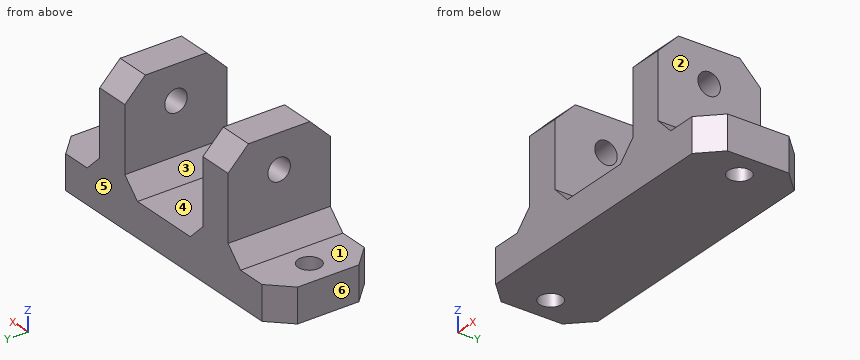
```python
from build123d import *

# Parameters (mm, degrees)
SKETCH_W        = 90
SKETCH_H        = 30
PAD_DEPTH       = 10
SKETCH001_W     = 10
SKETCH001_H     = 30
PAD001_DEPTH    = 30
CHAMFER_SIZE    = 6
SKETCH002_R     = 3.3
HOLE_DEPTH      = 58.01716
HOLE_TIPS_R     = 3.3
CHAMFER001_SIZE = 5
SKETCH003_R     = 3.3
HOLE001_DEPTH   = 25


with BuildPart() as part:
    # Sketch → Pad (new body)
    with BuildSketch(Plane.XY):
        Rectangle(SKETCH_W, SKETCH_H)
    extrude(amount=PAD_DEPTH)

    # Sketch001 → Pad001 (join)
    with BuildSketch(Plane.XY.offset(10)):
        with Locations((20.5, 0)):
            Rectangle(SKETCH001_W, SKETCH001_H)
        with Locations((-20.5, 0)):
            Rectangle(SKETCH001_W, SKETCH001_H)
    extrude(amount=PAD001_DEPTH)

    # Chamfer
    chamfer_edges = [part.edges().sort_by_distance(p)[0] for p in [
        (-45, 15, 5),
        (-45, -15, 5),
        (-20.5, 15, 40),
        (-20.5, -15, 40),
        (20.5, 15, 40),
        (45, 15, 5),
        (20.5, -15, 40),
        (45, -15, 5),
    ]]
    chamfer(chamfer_edges, length=CHAMFER_SIZE)

    # Sketch002 (on Face15 of Chamfer) → Hole (cut)
    with BuildSketch(Plane(origin=(-25.5, 0, 0), x_dir=(0, -1, 0), z_dir=(-1, 0, 0))):
        with Locations((0, 30)):
            Circle(SKETCH002_R)
    extrude(amount=-HOLE_DEPTH, mode=Mode.SUBTRACT)

    # Hole tips → Hole tip 1 section 0
    with BuildSketch(Plane(origin=(32.51716, 0, 0), x_dir=(0, -1, 0), z_dir=(-1, 0, 0)), mode=Mode.PRIVATE) as hole_tip_1_s0:
        with Locations((0, 30)):
            Circle(HOLE_TIPS_R)
    loft([hole_tip_1_s0.sketch, Vertex(34.5, 0, 30)], mode=Mode.SUBTRACT)

    # Chamfer001
    chamfer001_edges = [part.edges().sort_by_distance(p)[0] for p in [
        (25.5, 0, 10),
        (-15.5, 0, 10),
        (-25.5, 0, 10),
        (15.5, 0, 10),
    ]]
    chamfer(chamfer001_edges, length=CHAMFER001_SIZE)

    # Sketch003 (on Face2 of Chamfer001) → Hole001 (cut)
    with BuildSketch(Plane.XY.offset(10)):
        with Locations((-37.5, 0)):
            Circle(SKETCH003_R)
        with Locations((37.5, 0)):
            Circle(SKETCH003_R)
    extrude(amount=-HOLE001_DEPTH, mode=Mode.SUBTRACT)


solid = part.part
```
The model under review builds one solid part; all positions refer to its coordinate system, in mm. Face numbers are marked on the shaded views. A direction names the side the tool comes from. Round coordinates to 2 decimals unless told otherwise and drop trailing zeros. Loops run counter-clockwise (first coordinate to the right, second up) from the corner with the lowest first, then second, coordinate; pieces in that order, holes last. Notation, with made-up numbers: (43.25, -32) -> (70.25, -32) arc R21 cw to (70.25, -15) -> close; hole circle Ø9 at (83, -25.5). An arc over 180 degrees is marked (long way). Answer in a Markdown table with one row per item.
1) Consider section A-A, the plane x = 37.5. Write out the cut boundary in (y, z).
Taken from the geometry:
| item | result |
|---|---|
| outline | (-15, 0) -> (-3.3, 0) -> (-3.3, 10) -> (-15, 10) -> close; (3.3, 0) -> (15, 0) -> (15, 10) -> (3.3, 10) -> close |
2) Draft analysis for pull direction X (two halves, no side actions). For the marked faces 4, 5 and 6, state which applies: pulls with the +X half, pulls with the -X half, needs draft (parallel to the pull), parting line crosses it, or undercut.
Taken from the geometry:
| item | result |
|---|---|
| face 4 | undercut |
| face 5 | needs draft |
| face 6 | pulls with the -X half |
3) Wall thickness on line 1 along X through (y, z) = (0, 34.5); line 2 along Y through (x, z) = (-37.5, 7); line 3 along Z through (x, y) = (-20, 0): over which ranges is each line inside the solid? List them lowest first.
Taken from the geometry:
| item | result |
|---|---|
| line 1 | x = -25.5 to -15.5, 15.5 to 25.5 |
| line 2 | y = -15 to -3.3, 3.3 to 15 |
| line 3 | z = 0 to 26.7, 33.3 to 40 |
4) For pin 1 Ø17 at (x, y) = (1, -5) entering from +Z; pin 2 Ø12.5 at (y, z) = (7, 21.5) entering from +X; pin 3 Ø12.5 at (y, z) = (-4, 31.5) entering from -X, all flat-tipped, find the tip position at first contact; note any pin that passes through.
Taken from the geometry:
| item | result |
|---|---|
| pin 1 | stops at z = 10 |
| pin 2 | stops at x = 25.5 |
| pin 3 | stops at x = -25.5 |
5) Tool access review of the marked faces 1, 2 and 3: name each direction out of +Z, -Z, +X, -X, +Y, -Y from which nothing blocks a thin tool from reaching the whole face with its end or side.
Taken from the geometry:
| item | result |
|---|---|
| face 1 | +Z, -X, +Y, -Y |
| face 2 | +Z, +X, +Y, -Y |
| face 3 | +Z, +Y, -Y |
6) Consider section D-D, the plane y = 0. Count the separate pieces of the cut face and the enclosed holes in it, plus the area to 3 significant figures.
Taken from the geometry:
| item | result |
|---|---|
| separate pieces | 5 |
| enclosed holes | 0 |
| area | 1,290 mm² |
7) Consider section C-C, the plane z = 30. Write out the cut boundary in (x, y), plus the area to 3 significant figures.
Taken from the geometry:
| item | result |
|---|---|
| outline | (-25.5, -15) -> (-15.5, -15) -> (-15.5, -3.3) -> (-25.5, -3.3) -> close; (-25.5, 3.3) -> (-15.5, 3.3) -> (-15.5, 15) -> (-25.5, 15) -> close; (15.5, -15) -> (25.5, -15) -> (25.5, -3.3) -> (15.5, -3.3) -> close; (15.5, 3.3) -> (25.5, 3.3) -> (25.5, 15) -> (15.5, 15) -> close |
| area | 468 mm² |
8) Consider section B-B, the plane z = 11. Write out the cut boundary in (x, y), plus the area to 3 significant figures.
Taken from the geometry:
| item | result |
|---|---|
| outline | (-29.5, -15) -> (-11.5, -15) -> (-11.5, 15) -> (-29.5, 15) -> close; (11.5, -15) -> (29.5, -15) -> (29.5, 15) -> (11.5, 15) -> close |
| area | 1,080 mm² |
